Can you work these out from the drawing? Everything is in mm from the part's minimum corner. Round coordinates to 2 decimals unless told otherwise and drop trailing zeros. Write each loop counter-clockwise with the first axis right and the second up, starting at its lowest first coordinate (ties: lowest second). Pieces come first, ordered by that corner, then holes. Notation, with made-up numbers: (-25.75, 68.25) - (13.25, 68.25) arc R11 ccw to (13.25, 79.25) - close; hole circle Ø4 at (-35, -8.5). An arc over 180 degrees is marked (long way). One line per item, written item: value. Start each with the question number.
Item 1: For P1, Ø6, axis at x = 24.5, y = 20.5, coming from the -Z side, with a flat end and sliding along its axis, tell me the tip position at first contact or that it passes through.
Item 2: Imagine slicing it at A-A, the plane x = 34. Please give me the cut outline in (y, z).
Item 3: Imagine slicing it at B-B, the plane y = 62. Please give me the cut outline in (x, z).
Item 4: If I drill on line 1 (Y direction, x = 34, z = 4); line 2 (X direction, y = 4, z = 5.75); line 3 (Y direction, x = 33.5, z = 2.25), over which ranges is the centre line in solid material (lowest first)?
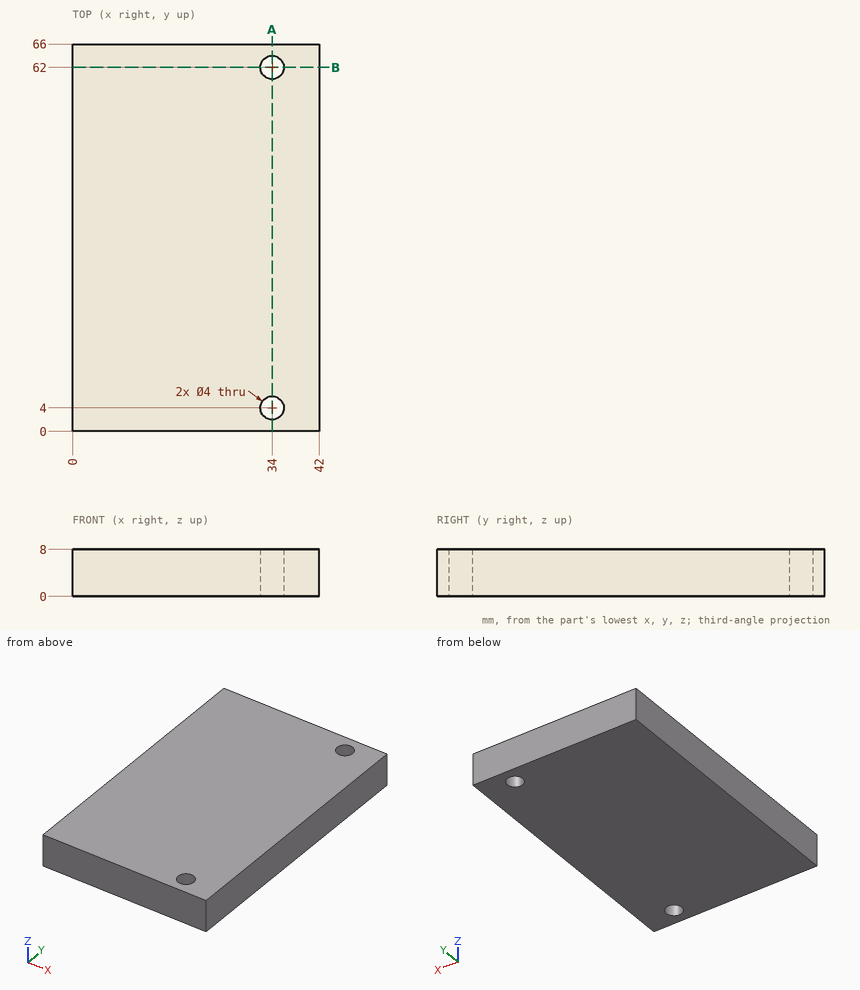
Values follow:
1. P1: stops at z = 0
2. outline: (0, 0) - (2, 0) - (2, 8) - (0, 8) - close; (6, 0) - (60, 0) - (60, 8) - (6, 8) - close; (64, 0) - (66, 0) - (66, 8) - (64, 8) - close
3. outline: (0, 0) - (32, 0) - (32, 8) - (0, 8) - close; (36, 0) - (42, 0) - (42, 8) - (36, 8) - close
4. line 1: y = 0 to 2, 6 to 60, 64 to 66
4. line 2: x = 0 to 32, 36 to 42
4. line 3: y = 0 to 2.06, 5.94 to 60.06, 63.94 to 66
